Design review of the part built by this model. Coordinates are the model's own, in mm. Face numbers are marked on the shaded views. Give positions to 0.01 mm unless a question says otherwise; leave off trailing zeros. Write each loop counter-clockwise with the first axis right and the second up, starting at its lowest first coordinate (ties: lowest second). Pieces come first, ordered by that corner, then holes.
```python
from build123d import *

# Parameters (mm, degrees)
F0_R     = 1.651
F1_DEPTH = 3.302
F2_R     = 3.175
F2_R_2   = 1.651
F3_DEPTH = 1.5748
F5_DEPTH = 15.875
F7_DEPTH = 14.2875


with BuildPart() as f1:
    # F0 (on Top) → F1 (new body)
    with BuildSketch(Plane.XY):
        with BuildLine():
            ThreePointArc((22.315054, -4.7625), (27.077554, 0), (22.315054, 4.7625))
            Line((22.315054, 4.7625), (22.315054, 8.5471))
            Line((22.315054, 8.5471), (-22.465146, 9.7536))
            Line((-22.465146, 9.7536), (-22.465146, 4.135386))
            ThreePointArc((-22.465146, 4.135386), (-24.865446, 0), (-22.465146, -4.135386))
            Line((-22.465146, -4.135386), (-22.465146, -9.7536))
            Line((-22.465146, -9.7536), (22.315054, -8.5471))
            Line((22.315054, -8.5471), (22.315054, -4.7625))
        make_face()
        with Locations((-20.102946, 0)):
            Circle(F0_R, mode=Mode.SUBTRACT)
        with Locations((22.315054, 0)):
            Circle(F0_R, mode=Mode.SUBTRACT)
    extrude(amount=F1_DEPTH)

    # F2 (on face) → F3 (cut)
    with BuildSketch(Plane.XY.offset(3.302)):
        with Locations((-20.102946, 0)):
            Circle(F2_R)
        with Locations((-20.102946, 0)):
            Circle(F2_R_2, mode=Mode.SUBTRACT)
        with Locations((22.315054, 0)):
            Circle(F2_R)
        with Locations((22.315054, 0)):
            Circle(F2_R_2, mode=Mode.SUBTRACT)
    extrude(amount=-F3_DEPTH, mode=Mode.SUBTRACT)

    # F4 (on Right) → F5 (join, symmetric)
    with BuildSketch(Plane.YZ):
        with BuildLine():
            ThreePointArc((7.9375, 3.302), (0, 6.477), (-7.9375, 3.302))
            Line((-7.9375, 3.302), (7.9375, 3.302))
        make_face()
    extrude(amount=F5_DEPTH, both=True)

    # F6 (on Right) → F7 (cut, symmetric)
    with BuildSketch(Plane.YZ):
        with BuildLine():
            ThreePointArc((6.35, 0), (0, 2.54), (-6.35, 0))
            Line((-6.35, 0), (6.35, 0))
        make_face()
    extrude(amount=F7_DEPTH, both=True, mode=Mode.SUBTRACT)


solid = f1.part
```
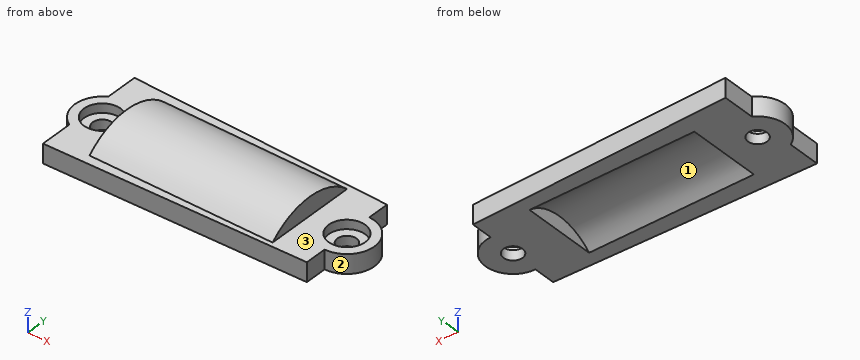
(1) Consider section A-A, the plane y = 0. Give the boundary of the cut face in (x, z) (1 decimal), then the cut area to 3 significant figures.
Resolved:
outline: (-24.9, 0) - (-21.8, 0) - (-21.8, 1.7) - (-23.3, 1.7) - (-23.3, 3.3) - (-24.9, 3.3) - close; (-18.5, 0) - (-14.3, 0) - (-14.3, 2.5) - (14.3, 2.5) - (14.3, 0) - (20.7, 0) - (20.7, 1.7) - (19.1, 1.7) - (19.1, 3.3) - (15.9, 3.3) - (15.9, 6.5) - (-15.9, 6.5) - (-15.9, 3.3) - (-16.9, 3.3) - (-16.9, 1.7) - (-18.5, 1.7) - close; (24, 0) - (27.1, 0) - (27.1, 3.3) - (25.5, 3.3) - (25.5, 1.7) - (24, 1.7) - close
area: 168 mm2
(2) Clearance check with flat-ended pins moving along their axes: P1, Ø1, axis at x = -7.5, y = -2.5, coming from the +Z side; P2, Ø1.5, axis at x = -9, z = 4.5, coming from the -Y side; P3, Ø2.5, axis at y = -1, z = 5.5, coming from the +X side (3 decimals); P4, Ø10, axis at x = -20.1, y = 0, coming from the -Z side. State where each tip first meets the part, or that it passes through.
Resolved:
P1: stops at z = 6.3
P2: stops at y = -7.44
P3: stops at x = 15.875
P4: stops at z = 0
(3) Consider section C-C, the plane y = -5.5. Give the boundary of the cut face in (x, z) (1 decimal), then the cut area to 3 significant figures.
Resolved:
outline: (-22.5, 0) - (-14.3, 0) - (-14.3, 0.7) - (14.3, 0.7) - (14.3, 0) - (22.3, 0) - (22.3, 3.3) - (15.9, 3.3) - (15.9, 5.1) - (-15.9, 5.1) - (-15.9, 3.3) - (-22.5, 3.3) - close
area: 184 mm2
(4) Consider section B-B, the plane z = 0.5. Give the boundary of the cut face in (x, y) (1 decimal).
Resolved:
outline: (-22.5, -9.8) - (22.3, -8.5) - (22.3, -4.8) arc R4.8 ccw to (22.3, 4.8) - (22.3, 8.5) - (-22.5, 9.8) - (-22.5, 4.1) arc R4.8 ccw to (-22.5, -4.1) - close; hole circle Ø3.3 at (-20.1, 0); hole (-14.3, -5.8) - (14.3, -5.8) - (14.3, 5.8) - (-14.3, 5.8) - close; hole circle Ø3.3 at (22.3, 0)
(5) To check wall thickness, follow L1, parallel to X at y = 1.5, z = 2; L2, parallel to Z at x = -17, y = -2.5; L3, parallel to X at y = -6, z = 0.5. State the ranges of each line that lie inside material, in increasing order.
Resolved:
L1: x = -24.62 to -22.9, -17.3 to -14.29, 14.29 to 19.52, 25.11 to 26.84
L2: z = 0 to 3.3
L3: x = -22.47 to 22.32
(6) Mouldability with a two-part tool opening along Y and no side actions: class the marked faces 1, 2 and 3 as pulls with the +Y half, pulls with the -Y half, needs draft (parallel to the pull), parting line crosses it, or undercut.
Resolved:
face 1: undercut
face 2: parting line crosses it
face 3: needs draft
